Model file for the job. Use its own axes, mm. A direction names the side the tool comes from. Coordinates: 2 decimals unless noted, no trailing zeros. Write each loop counter-clockwise with the first axis right and the second up, starting at its lowest first coordinate (ties: lowest second). Pieces come first, ordered by that corner, then holes. Notation, with made-up numbers: M 5.25,84 L 64.25,84 A10 cw 64.25,102 Z; hole C -20,11 d3. An arc over 180 degrees is marked long. One line per question, with ' | ' between items. Start each with the question number.
(1) Cut at B-B (x = -20). Write the cut outline in (y, z), plus the area to 3 significant figures.
(2) Flat gauge pin, fed straight in: pin 1 Ø4.5 at (x, z) = (1, -14) entering from +Y. Where does the tip first touch, or does it go through?
(3) Cut at A-A (y = -2.75). Write the cut outline in (x, z), plus the area to 3 significant figures.
(4) Wall check: probe 1 along X at (y, z) = (-1, 1.75); probe 2 along X at (y, z) = (1, -4.75); probe 3 along Y at (x, z) = (8, -12). Give the ranges that are in metal, low to high.
(5) Tool access for faces 5 (the face through (-20, -0.5, -5.1)), 6 (the face through (0, -2, -22.5)): list every direction of +Z, -Z, +X, -X, +Y, -Y with a clear straight run to the whole face (end or side of a thin tool).
(6) Two-plate mould, pull along X, no slides. Class faces 1 (the face through (29.14, -2.03, -21.6)), 2 (the face through (20, -0.5, 6.1)), 3 (the face through (-30, 0, -5)), 4 (the face through (0, 0, -17)): +X half, -X half, draft (parallel to the pull), parting line (faces both ways), or undercut.
(7) Cut at C-C (y = 2.25). Write the cut outline in (x, z), plus the area to 3 significant figures.
(8) Cut at D-D (z = -18.25). Write the cut outline in (x, y), plus the area to 3 significant figures.
from build123d import *

# Parameters (mm, degrees)
BOSS_EXTRUDE1_DEPTH = 3
SKETCH4_W           = 60
SKETCH4_H           = 30
BOSS_EXTRUDE2_DEPTH = 4
FILLET1_R           = 3
CUT_EXTRUDE1_DEPTH  = 8
BOSS_EXTRUDE3_DEPTH = 3


with BuildPart() as part:
    # Sketch2 → Boss-Extrude1 (new body)
    with BuildSketch(Plane(origin=(0, 0, 0), x_dir=(1, 0, 0), z_dir=(0, 1, 0))):
        with BuildLine():
            Line((-30, -7.5), (30, -7.5))
            Line((30, -7.5), (30, 11.664728706))
            ThreePointArc((30, 11.664728706), (29.572172135, 12.484862261), (28.654761905, 12.60324384))
            ThreePointArc((28.654761905, 12.60324384), (0, 7.5), (-28.654761905, 12.60324384))
            ThreePointArc((-28.654761905, 12.60324384), (-29.572172135, 12.484862261), (-30, 11.664728706))
            Line((-30, 11.664728706), (-30, -7.5))
        make_face()
    extrude(amount=BOSS_EXTRUDE1_DEPTH)

    # Sketch4 → Boss-Extrude2 (add)
    with BuildSketch(Plane.XZ):
        with Locations((0, -7.5)):
            Rectangle(SKETCH4_W, SKETCH4_H)
    extrude(amount=BOSS_EXTRUDE2_DEPTH)

    # Fillet1
    fillet1_edges = [part.edges().sort_by_distance(p)[0] for p in [
        (30, -2, -22.5),
        (30, -0.5, 7.5),
        (-30, -0.5, 7.5),
        (-30, -2, -22.5),
    ]]
    fillet(fillet1_edges, radius=FILLET1_R)

    # Sketch5 → Cut-Extrude1 (cut, through all)
    with BuildSketch(Plane(origin=(0, 3, 0), x_dir=(1, 0, 0), z_dir=(0, 1, 0))):
        with BuildLine():
            Line((1.6, 3.5), (1.6, -4.5))
            ThreePointArc((1.6, -4.5), (0, -6.1), (-1.6, -4.5))
            Line((-1.6, -4.5), (-1.6, 3.5))
            ThreePointArc((-1.6, 3.5), (0, 5.1), (1.6, 3.5))
        make_face()
        with BuildLine():
            Line((21.6, 3.5), (21.6, -4.5))
            ThreePointArc((21.6, -4.5), (20, -6.1), (18.4, -4.5))
            Line((18.4, -4.5), (18.4, 3.5))
            ThreePointArc((18.4, 3.5), (20, 5.1), (21.6, 3.5))
        make_face()
        with BuildLine():
            Line((-21.6, 3.5), (-21.6, -4.5))
            ThreePointArc((-21.6, -4.5), (-20, -6.1), (-18.4, -4.5))
            Line((-18.4, -4.5), (-18.4, 3.5))
            ThreePointArc((-18.4, 3.5), (-20, 5.1), (-21.6, 3.5))
        make_face()
    extrude(amount=-CUT_EXTRUDE1_DEPTH, mode=Mode.SUBTRACT)

    # Sketch6 → Boss-Extrude3 (add)
    with BuildSketch(Plane(origin=(0, 3, 0), x_dir=(1, 0, 0), z_dir=(0, 1, 0))):
        with BuildLine():
            Line((0, 7.5), (-28.824143961, 12.649144601))
            ThreePointArc((-28.824143961, 12.649144601), (-29.64192833, 12.43149335), (-30, 11.664728706))
            Line((-30, 11.664728706), (-30, -4.5))
            ThreePointArc((-30, -4.5), (-29.121320344, -6.621320344), (-27, -7.5))
            Line((-27, -7.5), (27, -7.5))
            ThreePointArc((27, -7.5), (29.121320344, -6.621320344), (30, -4.5))
            Line((30, -4.5), (30, 11.664728706))
            ThreePointArc((30, 11.664728706), (29.64192833, 12.43149335), (28.824143961, 12.649144601))
            Line((28.824143961, 12.649144601), (0, 7.5))
        make_face()
        with BuildLine():
            Line((-18.4, -4.5), (-18.4, 3.5))
            ThreePointArc((-18.4, 3.5), (-20, 5.1), (-21.6, 3.5))
            Line((-21.6, 3.5), (-21.6, -4.5))
            ThreePointArc((-21.6, -4.5), (-20, -6.1), (-18.4, -4.5))
        make_face(mode=Mode.SUBTRACT)
        with BuildLine():
            Line((1.6, -4.5), (1.6, 3.5))
            ThreePointArc((1.6, 3.5), (0, 5.1), (-1.6, 3.5))
            Line((-1.6, 3.5), (-1.6, -4.5))
            ThreePointArc((-1.6, -4.5), (0, -6.1), (1.6, -4.5))
        make_face(mode=Mode.SUBTRACT)
        with BuildLine():
            Line((21.6, -4.5), (21.6, 3.5))
            ThreePointArc((21.6, 3.5), (20, 5.1), (18.4, 3.5))
            Line((18.4, 3.5), (18.4, -4.5))
            ThreePointArc((18.4, -4.5), (20, -6.1), (21.6, -4.5))
        make_face(mode=Mode.SUBTRACT)
    extrude(amount=-BOSS_EXTRUDE3_DEPTH)


solid = part.part
Filled in:
1) outline: M -4,-22.5 L 0,-22.5 L 0,-11.07 L 3,-11.07 L 3,-5.1 L -4,-5.1 Z; M -4,6.1 L 3,6.1 L 3,7.5 L -4,7.5 Z | area: 97.3 mm²
2) pin 1: y = 0
3) outline: M -30,-19.5 A3 ccw -27,-22.5 L 27,-22.5 A3 ccw 30,-19.5 L 30,4.5 A3 ccw 27,7.5 L -27,7.5 A3 ccw -30,4.5 Z; hole M -21.6,-3.5 A1.6 ccw -18.4,-3.5 L -18.4,4.5 A1.6 ccw -21.6,4.5 Z; hole M -1.6,-3.5 A1.6 ccw 1.6,-3.5 L 1.6,4.5 A1.6 ccw -1.6,4.5 Z; hole M 18.4,-3.5 A1.6 ccw 21.6,-3.5 L 21.6,4.5 A1.6 ccw 18.4,4.5 Z | area: 1,690 mm²
4) probe 1: -30 to -21.6, -18.4 to -1.6, 1.6 to 18.4, 21.6 to 30 | probe 2: -30 to -21, -19 to -1, 1 to 19, 21 to 30 | probe 3: -4 to 0
5) face 5: +Y, -Y | face 6: -Z, +X, -X, +Y, -Y
6) face 1: +X half | face 2: undercut | face 3: -X half | face 4: undercut
7) outline: M -30,-11.66 A1 ccw -28.82,-12.65 L 0,-7.5 L 28.82,-12.65 A1 ccw 30,-11.66 L 30,4.5 A3 ccw 27,7.5 L -27,7.5 A3 ccw -30,4.5 Z; hole M -21.6,-3.5 A1.6 ccw -18.4,-3.5 L -18.4,4.5 A1.6 ccw -21.6,4.5 Z; hole M -1.6,-3.5 A1.6 ccw 1.6,-3.5 L 1.6,4.5 A1.6 ccw -1.6,4.5 Z; hole M 18.4,-3.5 A1.6 ccw 21.6,-3.5 L 21.6,4.5 A1.6 ccw 18.4,4.5 Z | area: 955 mm²
8) outline: M -30,-4 L 30,-4 L 30,0 L -30,0 Z | area: 240 mm²
